```python
from build123d import *

# Parameters (mm, degrees)
SKETCH_R        = 120
SKETCH_R_2      = 7
PAD_DEPTH       = 20
SKETCH001_R     = 115
SKETCH001_R_2   = 16
POCKET_DEPTH    = 8
SKETCH002_R     = 115
POCKET001_DEPTH = 6


with BuildPart() as part:
    # Sketch → Pad (new body)
    with BuildSketch(Plane.XY):
        Circle(SKETCH_R)
        Circle(SKETCH_R_2, mode=Mode.SUBTRACT)
    extrude(amount=PAD_DEPTH)

    # Sketch001 (on DatumPlane) → Pocket (cut)
    with BuildSketch(Plane.XY.offset(20)):
        Circle(SKETCH001_R)
        Circle(SKETCH001_R_2, mode=Mode.SUBTRACT)
    extrude(amount=-POCKET_DEPTH, mode=Mode.SUBTRACT)

    # Sketch002 (on DatumPlane) → Pocket001 (cut)
    with BuildSketch(Plane(origin=(0, 0, 0), x_dir=(1, 0, 0), z_dir=(0, 0, -1))):
        Circle(SKETCH002_R)
    extrude(amount=-POCKET001_DEPTH, mode=Mode.SUBTRACT)


solid = part.part
```
Check sheet for the modelled part. Datum: model origin and axes. Units: mm. A direction names the side the tool comes from. Round coordinates to 2 decimals unless told otherwise and drop trailing zeros. Loops run counter-clockwise (first coordinate to the right, second up) from the corner with the lowest first, then second, coordinate; pieces in that order, holes last. Notation, with made-up numbers: M 13.5,34.25 L 30.5,34.25 A7 ccw 30.5,47.25 Z; hole C 72,16 d2. An arc over 180 degrees is marked long. Answer as a JSON object with one key per item and string values.
1. Section check C-C (z = 17). Record the boundary of the cut face in (x, y).
Reply:
{"outline": "C 0,0 d240; C 0,0 d32; hole C 0,0 d230; hole C 0,0 d14"}
2. Gauge pin test, flat ends, axial feed: P1, Ø1, axis at y = -31.5, z = 9.5, coming from the -X side; P2, Ø4, axis at x = -52, z = 3, coming from the -Y side; P3, Ø2, axis at y = -33.5, z = 8.5, coming from the +X side; P4, Ø12.5, axis at x = 0, y = 0, coming from the +Z side. Record the tip position at first contact, or that the pin passes through.
Reply:
{"P1": "stops at x = -115.93", "P2": "stops at y = -109.09", "P3": "stops at x = 115.52", "P4": "passes through"}
3. Access from +Z, -Z, +X, -X, +Y, -Y to the whole of each face (thin tool, end or side, straight path). Record for faces 1 (the cylindrical face through (-24.93, 112.265, 2.958)), 2 (the cylindrical face through (6.466, -2.681, 12.902)), 3 (the flat face through (24, 2, 12)).
Reply:
{"face 1": "-Z", "face 2": "+Z, -Z", "face 3": "+Z"}
4. Mould release check, pull along Y, two halves, no side actions. Record for faces 4 (the cylindrical face through (-3.47, -15.62, 16.06)), 5 (the flat face through (24, -2, 6)), 6 (the flat face through (8, -115, 20)), 7 (the cylindrical face through (-119.884, 5.276, 9.86)): pulls with the +Y half, pulls with the -Y half, needs draft (parallel to the pull), parting line crosses it, or undercut.
Reply:
{"face 4": "undercut", "face 5": "undercut", "face 6": "needs draft", "face 7": "parting line crosses it"}
5. Section check D-D (y = -32.5). Record the boundary of the cut face in (x, z), plus the area to 3 significant figures.
Reply:
{"outline": "M -115.52,0 L -110.31,0 L -110.31,6 L 110.31,6 L 110.31,0 L 115.52,0 L 115.52,20 L 110.31,20 L 110.31,12 L -110.31,12 L -110.31,20 L -115.52,20 Z", "area": "1,530 mm²"}
6. Scan lines: line 1 (Y direction, x = 0, z = 18.25); line 2 (Y direction, x = 0, z = 3.65); line 3 (Y direction, x = 0, z = 11.5). Record each from-to range of solid material in increasing order.
Reply:
{"line 1": "y = -120 to -115, -16 to -7, 7 to 16, 115 to 120", "line 2": "y = -120 to -115, 115 to 120", "line 3": "y = -120 to -7, 7 to 120"}
7. Section check A-A (x = 0). Record the boundary of the cut face in (y, z).
Reply:
{"outline": "M -120,0 L -115,0 L -115,6 L -7,6 L -7,20 L -16,20 L -16,12 L -115,12 L -115,20 L -120,20 Z; M 7,6 L 115,6 L 115,0 L 120,0 L 120,20 L 115,20 L 115,12 L 16,12 L 16,20 L 7,20 Z"}
